```python
from build123d import *

# Parameters (mm, degrees)
SKETCH1_R             = 3.75
SKETCH1_R_2           = 1.75
BOSS_EXTRUDE1_DEPTH   = 3
CHAMFER1_SIZE         = 0.4
CHAMFER1_SIZE2        = 0.230940108
CHAMFER1_PART_2_SIZE  = 0.4
CHAMFER1_PART_2_SIZE2 = 0.230940108


with BuildPart() as part:
    # Sketch1 → Boss-Extrude1 (new body)
    with BuildSketch(Plane(origin=(0, 0, 0), x_dir=(1, 0, 0), z_dir=(0, 1, 0))):
        Circle(SKETCH1_R)
        Circle(SKETCH1_R_2, mode=Mode.SUBTRACT)
    extrude(amount=BOSS_EXTRUDE1_DEPTH)

    # Chamfer1
    chamfer1_edges = [part.edges().sort_by_distance(p)[0] for p in [
        (-3.75, 0, 0),
    ]]
    chamfer1_side = [part.faces().sort_by_distance(p)[0] for p in [
        (-3.643933983, 0, 0),
    ]]
    chamfer(chamfer1_edges, length=CHAMFER1_SIZE, length2=CHAMFER1_SIZE2, reference=chamfer1_side[0])

    # Chamfer1 part 2
    chamfer1_part_2_edges = [part.edges().sort_by_distance(p)[0] for p in [
        (-3.75, 3, 0),
    ]]
    chamfer1_part_2_side = [part.faces().sort_by_distance(p)[0] for p in [
        (-3.75, 1.5, 0),
    ]]
    chamfer(chamfer1_part_2_edges, length=CHAMFER1_PART_2_SIZE, length2=CHAMFER1_PART_2_SIZE2, reference=chamfer1_part_2_side[0])


solid = part.part
```
Input: part model. Units: mm. Frame: model coordinates. Round coordinates to 2 decimals unless told otherwise and drop trailing zeros. Order: outer loops, then holes, each group sorted by start corner. A loop starts at its lowest first (then second) coordinate and runs counter-clockwise, first axis right, second up. Notation, with made-up numbers: (-19, 8) - (14, 8) arc R9 cw to (14, 25) - close; hole circle Ø3 at (44, 15). An arc over 180 degrees is marked (long way). Answer in a Markdown table with one row per item.
Item 1: Line query: line 1 (Z direction, x = 0, y = 1.35); line 2 (X direction, y = 2.75, z = 1). Output: solid intervals per line, ascending.
Model answer:
| item | result |
|---|---|
| line 1 | z = -3.75 to -1.75, 1.75 to 3.75 |
| line 2 | x = -3.52 to -1.44, 1.44 to 3.52 |
Item 2: Section query A-A (x = 0). Return the cut outline in (y, z).
Model answer:
| item | result |
|---|---|
| outline | (0, -3.35) - (0.23, -3.75) - (2.6, -3.75) - (3, -3.52) - (3, -1.75) - (0, -1.75) - close; (0, 1.75) - (3, 1.75) - (3, 3.52) - (2.6, 3.75) - (0.23, 3.75) - (0, 3.35) - close |
Item 3: Section query B-B (z = 0). Return the cut outline in (x, y), then the cut area to 3 significant figures.
Model answer:
| item | result |
|---|---|
| outline | (-3.75, 0.23) - (-3.35, 0) - (-1.75, 0) - (-1.75, 3) - (-3.52, 3) - (-3.75, 2.6) - close; (1.75, 0) - (3.35, 0) - (3.75, 0.23) - (3.75, 2.6) - (3.52, 3) - (1.75, 3) - close |
| area | 11.8 mm² |
Item 4: Section query C-C (y = 2.1). Return the cut outline in (x, z), then the cut area to 3 significant figures.
Model answer:
| item | result |
|---|---|
| outline | circle Ø7.5 at (0, 0); hole circle Ø3.5 at (0, 0) |
| area | 34.6 mm² |
